from build123d import *

# Parameters (mm, degrees)
CROQUIS1_W               = 108
CROQUIS1_H               = 71
SALIENTE_EXTRUIR1_DEPTH  = 1.5
CROQUIS2_W               = 12
CROQUIS2_H               = 3
CROQUIS2_W_2             = 8
CORTAR_EXTRUIR1_DEPTH    = 3
CROQUIS6_W               = 3
CROQUIS6_H               = 14
CROQUIS6_H_2             = 8
CORTAR_EXTRUIR3_DEPTH    = 3
CROQUIS7_R               = 1.5
CROQUIS7_R_2             = 3
CROQUIS7_R_3             = 6.5
CROQUIS7_W               = 3.259373519
CROQUIS7_H               = 6.723882433
CORTAR_EXTRUIR4_DEPTH    = 23
CROQUIS8_W               = 8
CROQUIS8_H               = 3
SALIENTE_EXTRUIR2_DEPTH  = 3
REDONDEO2_R              = 3
CROQUIS9_R               = 1.5
CORTAR_EXTRUIR5_DEPTH    = 3
REDONDEO2_OF_SIMETR_A1_R = 3


with BuildPart() as part:
    # Croquis1 → Saliente-Extruir1 (new, symmetric)
    with BuildSketch(Plane(origin=(0, 0, 0), x_dir=(0, 0, -1), z_dir=(1, 0, 0))):
        Rectangle(CROQUIS1_W, CROQUIS1_H)
    extrude(amount=SALIENTE_EXTRUIR1_DEPTH, both=True)

    # Croquis2 → Cortar-Extruir1 (cut)
    with BuildSketch(Plane.ZY.offset(1.5)):
        with Locations((-48, -34)):
            Rectangle(CROQUIS2_W, CROQUIS2_H)
        with Locations((-24, -34)):
            Rectangle(CROQUIS2_W_2, CROQUIS2_H)
        with Locations((-8, -34)):
            Rectangle(CROQUIS2_W_2, CROQUIS2_H)
        with Locations((8, -34)):
            Rectangle(CROQUIS2_W_2, CROQUIS2_H)
        with Locations((24, -34)):
            Rectangle(CROQUIS2_W_2, CROQUIS2_H)
        with Locations((48, -34)):
            Rectangle(CROQUIS2_W, CROQUIS2_H)
        with Locations((48, 34)):
            Rectangle(CROQUIS2_W, CROQUIS2_H)
        with Locations((24, 34)):
            Rectangle(CROQUIS2_W_2, CROQUIS2_H)
        with Locations((8, 34)):
            Rectangle(CROQUIS2_W_2, CROQUIS2_H)
        with Locations((-8, 34)):
            Rectangle(CROQUIS2_W_2, CROQUIS2_H)
        with Locations((-24, 34)):
            Rectangle(CROQUIS2_W_2, CROQUIS2_H)
        with Locations((-48, 34)):
            Rectangle(CROQUIS2_W, CROQUIS2_H)
    extrude(amount=-CORTAR_EXTRUIR1_DEPTH, mode=Mode.SUBTRACT)

    # Croquis6 → Cortar-Extruir3 (cut)
    with BuildSketch(Plane.ZY.offset(1.5)):
        with Locations((52.5, -28.5)):
            Rectangle(CROQUIS6_W, CROQUIS6_H)
        with Locations((52.5, -6.5)):
            Rectangle(CROQUIS6_W, CROQUIS6_H_2)
        with Locations((52.5, 6.5)):
            Rectangle(CROQUIS6_W, CROQUIS6_H_2)
        with Locations((52.5, 28.5)):
            Rectangle(CROQUIS6_W, CROQUIS6_H)
    extrude(amount=-CORTAR_EXTRUIR3_DEPTH, mode=Mode.SUBTRACT)

    # Croquis7 → Cortar-Extruir4 (cut)
    with BuildSketch(Plane.ZY.offset(1.5)):
        with Locations((-3.2, -11.5)):
            Circle(CROQUIS7_R)
        with Locations((-3.2, -29)):
            Circle(CROQUIS7_R)
        with Locations((-13, -20.25)):
            Circle(CROQUIS7_R_2)
        with Locations((-23.8, -20.25)):
            Circle(CROQUIS7_R_3)
        with Locations((8.36450747, -20.229697644)):
            Rectangle(CROQUIS7_W, CROQUIS7_H)
    extrude(amount=-CORTAR_EXTRUIR4_DEPTH, mode=Mode.SUBTRACT)

    # Croquis8 → Saliente-Extruir2 (add)
    with BuildSketch(Plane.ZY.offset(1.5)):
        with Locations((16, 37)):
            Rectangle(CROQUIS8_W, CROQUIS8_H)
    saliente_extruir2 = extrude(amount=-SALIENTE_EXTRUIR2_DEPTH)

    # Redondeo2
    redondeo2_edges = [part.edges().sort_by_distance(p)[0] for p in [
        (0, 38.5, 12),
        (0, 38.5, 20),
    ]]
    fillet(redondeo2_edges, radius=REDONDEO2_R)

    # Croquis9 → Cortar-Extruir5 (cut)
    with BuildSketch(Plane.ZY.offset(1.5)):
        with Locations((16, 34)):
            Circle(CROQUIS9_R)
    cortar_extruir5 = extrude(amount=-CORTAR_EXTRUIR5_DEPTH, mode=Mode.SUBTRACT)

    # Simetría1: Saliente-Extruir2, Cortar-Extruir5 across plane
    add(saliente_extruir2.mirror(Plane.ZX))
    add(cortar_extruir5.mirror(Plane.ZX), mode=Mode.SUBTRACT)

    # Redondeo2 of Simetría1
    redondeo2_of_simetr_a1_edges = [part.edges().sort_by_distance(p)[0] for p in [
        (0, -38.5, 12),
        (0, -38.5, 20),
    ]]
    fillet(redondeo2_of_simetr_a1_edges, radius=REDONDEO2_OF_SIMETR_A1_R)


solid = part.part
Can you work these out from the model? Positions are in its coordinate system, mm. A direction names the side the tool comes from. Coordinates: 2 decimals unless noted, no trailing zeros. Write each loop counter-clockwise with the first axis right and the second up, starting at its lowest first coordinate (ties: lowest second). Pieces come first, ordered by that corner, then holes. Notation, with made-up numbers: (73.25, 76.25) -> (89.25, 76.25) arc R25 cw to (89.25, 101.25) -> close; hole circle Ø1 at (-39, 69). An arc over 180 degrees is marked (long way). Write item = value, one per line.
(1) Imagine slicing it at B-B (z = -14.5). Please give me the cut outline in (x, y), and give its area (3 significant figures).
Verdict:
outline = (-1.5, -35.5) -> (1.5, -35.5) -> (1.5, -22.85) -> (-1.5, -22.85) -> close; (-1.5, -17.65) -> (1.5, -17.65) -> (1.5, 35.5) -> (-1.5, 35.5) -> close
area = 197 mm^2
(2) If I drill on probe 1 along Y at (x, z) = (0.55, 16); probe 2 along Y at (x, z) = (-0.8, 26); probe 3 along Y at (x, z) = (-0.2, -13), over which ranges is the centre line in solid material (lowest first)?
Verdict:
probe_1 = -38.5 to -35.5, -32.5 to 32.5, 35.5 to 38.5
probe_2 = -32.5 to 32.5
probe_3 = -35.5 to -23.25, -17.25 to 35.5
(3) Imagine slicing it at A-A (y = 34). Please give me the cut outline in (x, z).
Verdict:
outline = (-1.5, -42) -> (1.5, -42) -> (1.5, -28) -> (-1.5, -28) -> close; (-1.5, -20) -> (1.5, -20) -> (1.5, -12) -> (-1.5, -12) -> close; (-1.5, -4) -> (1.5, -4) -> (1.5, 4) -> (-1.5, 4) -> close; (-1.5, 12) -> (1.5, 12) -> (1.5, 14.5) -> (-1.5, 14.5) -> close; (-1.5, 17.5) -> (1.5, 17.5) -> (1.5, 20) -> (-1.5, 20) -> close; (-1.5, 28) -> (1.5, 28) -> (1.5, 42) -> (-1.5, 42) -> close
(4) Thinking about a two-plate mould opening in Z: for faces 4 (the face through (0, 34, -4)), 5 (the face through (0, 32.5, 8)), 6 (the face through (0.02, -37.6, 12.86)), 7 (the face through (0, -38.5, 16)), which applies, +Z half, -Z half, draft (parallel to the pull), parting line (faces both ways), or undercut?
Verdict:
face_4 = undercut
face_5 = undercut
face_6 = -Z half
face_7 = draft
(5) Imagine slicing it at D-D (z = 36). Please give me the cut outline in (x, y), and give its area (3 significant figures).
Verdict:
outline = (-1.5, -35.5) -> (1.5, -35.5) -> (1.5, 35.5) -> (-1.5, 35.5) -> close
area = 213 mm^2
(6) Imagine slicing it at C-C (x = 1). State how many separate pieces and enclosed holes the cut face has, and give its area (3 significant figures).
Verdict:
separate_pieces = 1
enclosed_holes = 7
area = 7,050 mm^2
(7) On a 3-axis mill with a long thin cutter (end or side, diameter ignored), from which of +Z, -Z, +X, -X, +Y, -Y can I reach the whole of each face in a straight line? I mean faces 1 (the face through (0, -35.5, -16)), 2 (the face through (0, 10.5, 52)), 3 (the face through (0, 34, -28)). Say none if no direction works.
Verdict:
face_1 = -Z, +X, -X, -Y
face_2 = +Z, +X, -X
face_3 = +X, -X, +Y
(8) For pin 1 (0.9 mm diameter, centred on x = 0, y = 34, fed in from +Z); pin 2 (0.9 mm diameter, centred on x = -0.5, z = -25.5, fed in from -Y); pin 3 (0.9 mm diameter, centred on x = 0.5, z = 52.5, fed in from -Y); pin 4 (5 mm diameter, centred on y = -20.25, z = -13, fed in from +X), each with a flat end and sliding along its axis, tell me the tip position at first contact or that it passes through.
Verdict:
pin_1 = 42
pin_2 = -32.5
pin_3 = -21.5
pin_4 = through
